Work out the finished part from the listing and answer in its coordinate system (mm). A direction names the side the tool comes from. Round coordinates to 2 decimals unless told otherwise and drop trailing zeros. Order: outer loops, then holes, each group sorted by start corner. A loop starts at its lowest first (then second) coordinate and runs counter-clockwise, first axis right, second up. Notation, with made-up numbers: M 48,-0.5 L 87,-0.5 A34 cw 87,31.5 Z; hole C 49,87.25 d7. An arc over 180 degrees is marked long. Return JSON: item names as keys, results as strings.
from build123d import *

# Parameters (mm, degrees)
SKETCH1_W           = 200
SKETCH1_H           = 140
BOSS_EXTRUDE1_DEPTH = 2
CUT_EXTRUDE1_DEPTH  = 123.131077126
FILLET1_R           = 5


with BuildPart() as part:
    # Sketch1 → Boss-Extrude1 (new, symmetric)
    with BuildSketch(Plane(origin=(0, 0, 0), x_dir=(1, 0, 0), z_dir=(0, 1, 0))):
        Rectangle(SKETCH1_W, SKETCH1_H)
    extrude(amount=BOSS_EXTRUDE1_DEPTH, both=True)

    # Sketch2 → Cut-Extrude1 (cut, through all)
    with BuildSketch(Plane(origin=(0, 2, 0), x_dir=(1, 0, 0), z_dir=(0, 1, 0))):
        with BuildLine():
            Line((-82, 60), (-82, 50))
            ThreePointArc((-82, 50), (-85, 47), (-88, 50))
            Line((-88, 50), (-88, 60))
            ThreePointArc((-88, 60), (-85, 63), (-82, 60))
        make_face()
        with BuildLine():
            Line((82, 60), (82, 50))
            ThreePointArc((82, 50), (85, 47), (88, 50))
            Line((88, 50), (88, 60))
            ThreePointArc((88, 60), (85, 63), (82, 60))
        make_face()
        with BuildLine():
            Line((82, -60), (82, -50))
            ThreePointArc((82, -50), (85, -47), (88, -50))
            Line((88, -50), (88, -60))
            ThreePointArc((88, -60), (85, -63), (82, -60))
        make_face()
        with BuildLine():
            Line((-82, -60), (-82, -50))
            ThreePointArc((-82, -50), (-85, -47), (-88, -50))
            Line((-88, -50), (-88, -60))
            ThreePointArc((-88, -60), (-85, -63), (-82, -60))
        make_face()
    extrude(amount=-CUT_EXTRUDE1_DEPTH, mode=Mode.SUBTRACT)

    # Fillet1
    fillet1_edges = [part.edges().sort_by_distance(p)[0] for p in [
        (100, 0, 70),
        (-100, 0, 70),
        (-100, 0, -70),
        (100, 0, -70),
    ]]
    fillet(fillet1_edges, radius=FILLET1_R)


solid = part.part
Item 1: Find section A-A (x = -85). Determine the outline of the cut face in (y, z).
Output:
{"outline": "M -2,-70 L 2,-70 L 2,-63 L -2,-63 Z; M -2,-47 L 2,-47 L 2,47 L -2,47 Z; M -2,63 L 2,63 L 2,70 L -2,70 Z"}
Item 2: The mould has two halves that part along X. Classify faces 1 (the flat face through (-1, 2, -1)), 2 (the flat face through (88, 0, -55)), 3 (the flat face through (-100, 0, 1)): pulls with the +X half, pulls with the -X half, needs draft (parallel to the pull), parting line crosses it, or undercut.
Output:
{"face 1": "needs draft", "face 2": "undercut", "face 3": "pulls with the -X half"}
Item 3: Which of the six approach directions +Z, -Z, +X, -X, +Y, -Y give full straight-line access (tool end or side, diameter ignored) to faces 4 (the flat face through (-1, 0, 70)), 5 (the flat face through (-82, 0, -55))?
Output:
{"face 4": "+Z, +X, -X, +Y, -Y", "face 5": "+Y, -Y"}
Item 4: Consider line 1 along X through (y, z) = (-1.2, 61.5); line 2 along Z through (x, y) = (-87, -0.3); line 3 along X through (y, z) = (-0.7, 61). Determine where each line is inside the solid, lowest interval first. Write a range as [from, to].
Output:
{"line 1": "x = [-100, -87.6], [-82.4, 82.4], [87.6, 100]", "line 2": "z = [-70, -62.24], [-47.76, 47.76], [62.24, 70]", "line 3": "x = [-100, -87.83], [-82.17, 82.17], [87.83, 100]"}
